Could you check a few things on this drawing? It's one solid part, dimensions in mm from its lowest x, y, z. A direction names the side the tool comes from. Round coordinates to 2 decimals unless told otherwise and drop trailing zeros. Write each loop counter-clockwise with the first axis right and the second up, starting at its lowest first coordinate (ties: lowest second). Pieces come first, ordered by that corner, then holes. Notation, with made-up numbers: (9.25, 29) - (30.25, 29) arc R21 ccw to (30.25, 45) - close; hole circle Ø8 at (-13, 36). An arc over 180 degrees is marked (long way). Use one line per item in the form item = value. Start each with the question number.
1. Will these pins go through, and if not, where does the flat tip stop? pin 1 (2 mm diameter, centred on x = 62, y = 6.5, fed in from +Z); pin 2 (4.5 mm diameter, centred on y = 7, z = 5.5, fed in from -X); pin 3 (1.2 mm diameter, centred on x = 24, y = 5, fed in from -Z).
2. I want a section at C-C, the plane z = 6.5. List the corners of the cut face in (x, y) for me.
3. Which directions (+Z, -Z, +X, -X, +Y, -Y) give clear straight access to the entire face, cutting with the end or side of a thin tool? Please do the marked faces 1 and 2.
4. We'd pull the mould along X, two halves only. Please class the marked faces 3, 4 and 5: +X half, -X half, draft (parallel to the pull), parting line (faces both ways), or undercut.
5. If I drill on line 1 along Y through (x, z) = (24, 0.4); line 2 along X through (y, z) = (4, 2.5); line 3 along Z through (x, y) = (62, 4.5), over which ranges is the centre line in solid material (lowest first)?
6. I want a section at A-A, the plane x = 72. List the corners of the cut face in (y, z) for me, plus the area to 3 significant figures.
7. I want a section at B-B, the plane y = 5. List the corners of the cut face in (x, z) for me, plus the area to 3 significant figures.
8. I want a section at D-D, the plane x = 84.5. List the corners of the cut face in (y, z) for me, plus the area to 3 significant figures.
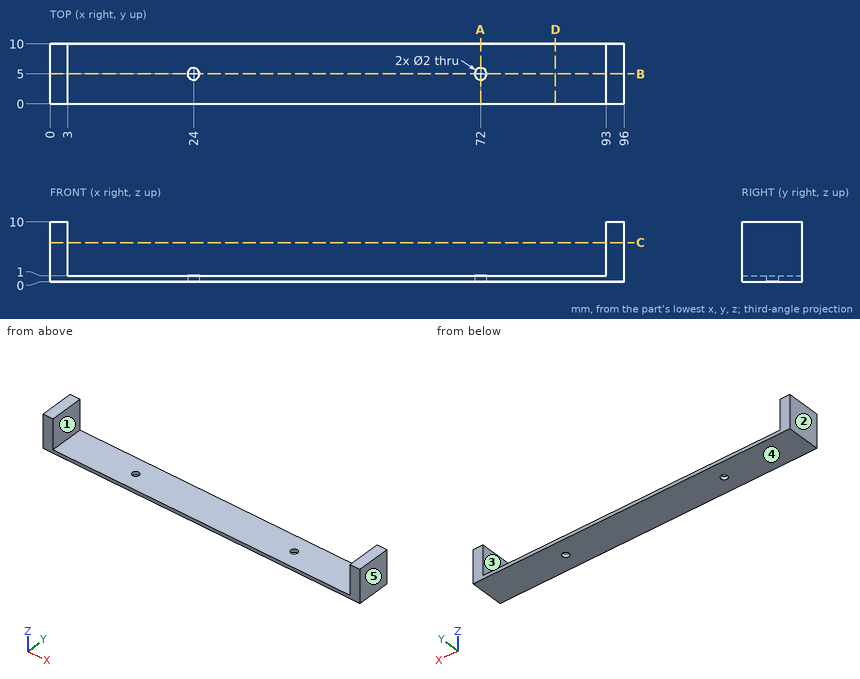
Model answer:
q1.pin_1 = 1
q1.pin_2 = 0
q1.pin_3 = through
q2.outline = (0, 0) - (3, 0) - (3, 10) - (0, 10) - close; (93, 0) - (96, 0) - (96, 10) - (93, 10) - close
q3.face_1 = +Z, +Y, -Y
q3.face_2 = +Z, -Z, -X, +Y, -Y
q4.face_3 = undercut
q4.face_4 = draft
q4.face_5 = +X half
q5.line_1 = 0 to 4, 6 to 10
q5.line_2 = 0 to 3, 93 to 96
q5.line_3 = 0 to 1
q6.outline = (0, 0) - (4, 0) - (4, 1) - (0, 1) - close; (6, 0) - (10, 0) - (10, 1) - (6, 1) - close
q6.area = 8.00 mm2
q7.outline = (0, 0) - (23, 0) - (23, 1) - (3, 1) - (3, 10) - (0, 10) - close; (25, 0) - (71, 0) - (71, 1) - (25, 1) - close; (73, 0) - (96, 0) - (96, 10) - (93, 10) - (93, 1) - (73, 1) - close
q7.area = 146 mm2
q8.outline = (0, 0) - (10, 0) - (10, 1) - (0, 1) - close
q8.area = 10.0 mm2
